Read the model definition and answer for the solid it produces. Units are mm, in the model's axes. A direction names the side the tool comes from. Coordinates: 2 decimals unless noted, no trailing zeros. Order: outer loops, then holes, each group sorted by start corner. A loop starts at its lowest first (then second) coordinate and runs counter-clockwise, first axis right, second up.
```python
from build123d import *

# Parameters (mm, degrees)
S_BOX1_W        = 30.8
S_BOX1_H        = 34.5
BOSS_1_DEPTH    = 2.5
S_BOX2_W        = 30.8
S_BOX2_H        = 34.5
BOSS_2_DEPTH    = 2.5
S_BOX3_W        = 2.5
S_BOX3_H        = 34.5
BOSS_3_DEPTH    = 51.4
S_BOX4_W        = 2.5
S_BOX4_H        = 34.5
BOSS_4_DEPTH    = 51.4
S_BOX5_W        = 30.8
S_BOX5_H        = 3
BOSS_5_DEPTH    = 51.4
S_BOX6_W        = 2.5
S_BOX6_H        = 34.5
BOSS_6_DEPTH    = 30.8
S_BOX7_W        = 2.5
S_BOX7_H        = 34.5
BOSS_7_DEPTH    = 30.8
S_BOX8_W        = 51.4
S_BOX8_H        = 34.5
BOSS_8_DEPTH    = 2.5
S_BOX9_W        = 51.4
S_BOX9_H        = 34.5
BOSS_9_DEPTH    = 2.5
S_BOX10_W       = 51.4
S_BOX10_H       = 3
BOSS_10_DEPTH   = 30.8
BOSS_11_DEPTH   = 34.5
S_CYL12_R       = 3.5
BOSS_12_DEPTH   = 7.7
S_HOLE13_R      = 10.5
HOLE_13_DEPTH   = 3.2
S_CUT14_W       = 19.4
S_CUT14_H       = 3.15
POCKET_14_DEPTH = 19.5
S_CUT15_W       = 16.4
S_CUT15_H       = 3.15
POCKET_15_DEPTH = 8.3
S_CUT16_W       = 7
S_CUT16_H       = 3.15
POCKET_16_DEPTH = 11
S_HOLE17_R      = 1.1
HOLE_17_DEPTH   = 3.2
S_HOLE18_R      = 1.1
HOLE_18_DEPTH   = 3.2
S_HOLE19_R      = 1.1
HOLE_19_DEPTH   = 3.2
S_HOLE20_R      = 1.1
HOLE_20_DEPTH   = 3.2
S_HOLE21_R      = 10.5
HOLE_21_DEPTH   = 3.2
S_CUT22_W       = 19.5
S_CUT22_H       = 3.15
POCKET_22_DEPTH = 19.4
S_CUT23_W       = 8.3
S_CUT23_H       = 3.15
POCKET_23_DEPTH = 16.4
S_CUT24_W       = 11
S_CUT24_H       = 3.15
POCKET_24_DEPTH = 7
S_HOLE25_R      = 1.1
HOLE_25_DEPTH   = 3.2
S_HOLE26_R      = 1.1
HOLE_26_DEPTH   = 3.2
S_HOLE27_R      = 1.1
HOLE_27_DEPTH   = 3.2
S_HOLE28_R      = 1.1
HOLE_28_DEPTH   = 3.2


with BuildPart() as part:
    # S_box1 → Boss_1 (new body)
    with BuildSketch(Plane.XY.offset(-38.2)):
        with Locations((0, -20.15)):
            Rectangle(S_BOX1_W, S_BOX1_H)
    extrude(amount=BOSS_1_DEPTH)



with BuildPart() as body_2:
    # S_box2 → Boss_2 (new body)
    with BuildSketch(Plane.XY.offset(10.7)):
        with Locations((0, -20.15)):
            Rectangle(S_BOX2_W, S_BOX2_H)
    extrude(amount=BOSS_2_DEPTH)


with BuildPart() as part_1:
    add(part.part)

    add(body_2.part)  # Boss_3 merges body 2
    # S_box3 → Boss_3 (add)
    with BuildSketch(Plane.XY.offset(-38.2)):
        with Locations((-14.15, -20.15)):
            Rectangle(S_BOX3_W, S_BOX3_H)
    extrude(amount=BOSS_3_DEPTH)

    # S_box4 → Boss_4 (add)
    with BuildSketch(Plane.XY.offset(-38.2)):
        with Locations((14.15, -20.15)):
            Rectangle(S_BOX4_W, S_BOX4_H)
    extrude(amount=BOSS_4_DEPTH)

    # S_box5 → Boss_5 (add)
    with BuildSketch(Plane.XY.offset(-38.2)):
        with Locations((0, -35.9)):
            Rectangle(S_BOX5_W, S_BOX5_H)
    extrude(amount=BOSS_5_DEPTH)

    # S_box6 → Boss_6 (add)
    with BuildSketch(Plane.XY.offset(-67.4)):
        with Locations((-11.95, -20.85)):
            Rectangle(S_BOX6_W, S_BOX6_H)
    extrude(amount=BOSS_6_DEPTH)



with BuildPart() as body_2_2:
    # S_box7 → Boss_7 (new body)
    with BuildSketch(Plane.XY.offset(-67.4)):
        with Locations((36.95, -20.85)):
            Rectangle(S_BOX7_W, S_BOX7_H)
    extrude(amount=BOSS_7_DEPTH)


with BuildPart() as part_2:
    add(part_1.part)

    add(body_2_2.part)  # Boss_8 merges body 2 2
    # S_box8 → Boss_8 (add)
    with BuildSketch(Plane.XY.offset(-67.4)):
        with Locations((12.5, -20.85)):
            Rectangle(S_BOX8_W, S_BOX8_H)
    extrude(amount=BOSS_8_DEPTH)

    # S_box9 → Boss_9 (add)
    with BuildSketch(Plane.XY.offset(-39.1)):
        with Locations((12.5, -20.85)):
            Rectangle(S_BOX9_W, S_BOX9_H)
    extrude(amount=BOSS_9_DEPTH)

    # S_box10 → Boss_10 (add)
    with BuildSketch(Plane.XY.offset(-67.4)):
        with Locations((12.5, -5.1)):
            Rectangle(S_BOX10_W, S_BOX10_H)
    extrude(amount=BOSS_10_DEPTH)

    # S_prism11 → Boss_11 (add)
    with BuildSketch(Plane(origin=(0, -37.4, 0), x_dir=(1, 0, 0), z_dir=(0, 1, 0))):
        with BuildLine():
            Line((-15.45, -10.75), (15.45, -10.75))
            Line((15.45, -10.75), (15.45, -11.2))
            ThreePointArc((15.45, -11.2), (13.6926, -15.4426), (9.45, -17.2))
            Line((9.45, -17.2), (-9.45, -17.2))
            ThreePointArc((-9.45, -17.2), (-13.6926, -15.4426), (-15.45, -11.2))
            Line((-15.45, -11.2), (-15.45, -10.75))
        make_face()
    extrude(amount=BOSS_11_DEPTH)

    # S_cyl12 → Boss_12 (add)
    with BuildSketch(Plane(origin=(0, -44.2, 0), x_dir=(1, 0, 0), z_dir=(0, 1, 0))):
        with Locations(Location((13, 17, 0), (0, 0, 46.708192407))):
            Circle(S_CYL12_R)
    extrude(amount=BOSS_12_DEPTH)

    # S_hole13 → Hole_13 (cut)
    with BuildSketch(Plane(origin=(0, -37.5, 0), x_dir=(1, 0, 0), z_dir=(0, 1, 0))):
        with Locations(Location((0, 0, 0), (0, 0, 90))):
            Circle(S_HOLE13_R)
    extrude(amount=HOLE_13_DEPTH, mode=Mode.SUBTRACT)

    # S_cut14 → Pocket_14 (cut)
    with BuildSketch(Plane.XY.offset(-30.4)):
        with Locations((0, -35.925)):
            Rectangle(S_CUT14_W, S_CUT14_H)
    extrude(amount=POCKET_14_DEPTH, mode=Mode.SUBTRACT)

    # S_cut15 → Pocket_15 (cut)
    with BuildSketch(Plane.XY.offset(-38.7)):
        with Locations((0, -35.925)):
            Rectangle(S_CUT15_W, S_CUT15_H)
    extrude(amount=POCKET_15_DEPTH, mode=Mode.SUBTRACT)

    # S_cut16 → Pocket_16 (cut)
    with BuildSketch(Plane.XY.offset(-11)):
        with Locations((0, -35.925)):
            Rectangle(S_CUT16_W, S_CUT16_H)
    extrude(amount=POCKET_16_DEPTH, mode=Mode.SUBTRACT)

    # S_hole17 → Hole_17 (cut)
    with BuildSketch(Plane(origin=(0, -37.5, 0), x_dir=(1, 0, 0), z_dir=(0, 1, 0))):
        with Locations(Location((-10.25, 8.3, 0), (0, 0, 90))):
            Circle(S_HOLE17_R)
    extrude(amount=HOLE_17_DEPTH, mode=Mode.SUBTRACT)

    # S_hole18 → Hole_18 (cut)
    with BuildSketch(Plane(origin=(0, -37.5, 0), x_dir=(1, 0, 0), z_dir=(0, 1, 0))):
        with Locations(Location((10.25, 8.3, 0), (0, 0, 90))):
            Circle(S_HOLE18_R)
    extrude(amount=HOLE_18_DEPTH, mode=Mode.SUBTRACT)

    # S_hole19 → Hole_19 (cut)
    with BuildSketch(Plane(origin=(0, -37.5, 0), x_dir=(1, 0, 0), z_dir=(0, 1, 0))):
        with Locations(Location((-10.25, 32.75, 0), (0, 0, 90))):
            Circle(S_HOLE19_R)
    extrude(amount=HOLE_19_DEPTH, mode=Mode.SUBTRACT)

    # S_hole20 → Hole_20 (cut)
    with BuildSketch(Plane(origin=(0, -37.5, 0), x_dir=(1, 0, 0), z_dir=(0, 1, 0))):
        with Locations(Location((10.25, 32.75, 0), (0, 0, 90))):
            Circle(S_HOLE20_R)
    extrude(amount=HOLE_20_DEPTH, mode=Mode.SUBTRACT)

    # S_hole21 → Hole_21 (cut)
    with BuildSketch(Plane(origin=(0, -6.7, 0), x_dir=(1, 0, 0), z_dir=(0, 1, 0))):
        with Locations(Location((0, 52, 0), (0, 0, 90))):
            Circle(S_HOLE21_R)
    extrude(amount=HOLE_21_DEPTH, mode=Mode.SUBTRACT)

    # S_cut22 → Pocket_22 (cut)
    with BuildSketch(Plane.XY.offset(-61.7)):
        with Locations((20.65, -5.075)):
            Rectangle(S_CUT22_W, S_CUT22_H)
    extrude(amount=POCKET_22_DEPTH, mode=Mode.SUBTRACT)

    # S_cut23 → Pocket_23 (cut)
    with BuildSketch(Plane.XY.offset(-60.2)):
        with Locations((34.55, -5.075)):
            Rectangle(S_CUT23_W, S_CUT23_H)
    extrude(amount=POCKET_23_DEPTH, mode=Mode.SUBTRACT)

    # S_cut24 → Pocket_24 (cut)
    with BuildSketch(Plane.XY.offset(-55.5)):
        with Locations((5.5, -5.075)):
            Rectangle(S_CUT24_W, S_CUT24_H)
    extrude(amount=POCKET_24_DEPTH, mode=Mode.SUBTRACT)

    # S_hole25 → Hole_25 (cut)
    with BuildSketch(Plane(origin=(0, -6.7, 0), x_dir=(1, 0, 0), z_dir=(0, 1, 0))):
        with Locations(Location((8.3, 62.25, 0), (0, 0, 90))):
            Circle(S_HOLE25_R)
    extrude(amount=HOLE_25_DEPTH, mode=Mode.SUBTRACT)

    # S_hole26 → Hole_26 (cut)
    with BuildSketch(Plane(origin=(0, -6.7, 0), x_dir=(1, 0, 0), z_dir=(0, 1, 0))):
        with Locations(Location((8.3, 41.75, 0), (0, 0, 90))):
            Circle(S_HOLE26_R)
    extrude(amount=HOLE_26_DEPTH, mode=Mode.SUBTRACT)

    # S_hole27 → Hole_27 (cut)
    with BuildSketch(Plane(origin=(0, -6.7, 0), x_dir=(1, 0, 0), z_dir=(0, 1, 0))):
        with Locations(Location((32.75, 62.25, 0), (0, 0, 90))):
            Circle(S_HOLE27_R)
    extrude(amount=HOLE_27_DEPTH, mode=Mode.SUBTRACT)

    # S_hole28 → Hole_28 (cut)
    with BuildSketch(Plane(origin=(0, -6.7, 0), x_dir=(1, 0, 0), z_dir=(0, 1, 0))):
        with Locations(Location((32.75, 41.75, 0), (0, 0, 90))):
            Circle(S_HOLE28_R)
    extrude(amount=HOLE_28_DEPTH, mode=Mode.SUBTRACT)


solid = part_2.part
```
1) A cutting plane is placed at D-D, the plane x = 0. Determine the outline of the cut face in (y, z), and give its area (3 significant figures).
A:
outline: (-38.1, -67.4) - (-3.6, -67.4) - (-3.6, -62.5) - (-6.6, -62.5) - (-6.6, -64.9) - (-38.1, -64.9) - close; (-38.1, -39.1) - (-6.6, -39.1) - (-6.6, -41.5) - (-3.6, -41.5) - (-3.6, -38.2) - (-2.9, -38.2) - (-2.9, -35.7) - (-34.35, -35.7) - (-34.35, -38.7) - (-37.5, -38.7) - (-37.5, -36.6) - (-38.1, -36.6) - close; (-37.4, 10.5) - (-34.4, 10.5) - (-34.4, 10.7) - (-2.9, 10.7) - (-2.9, 17.2) - (-37.4, 17.2) - close
area: 435 mm2
2) Flat-ended cylindrical pins translate along their axes: pin 1 Ø5 at (y, z) = (-30.5, -8.5) entering from -X; pin 2 Ø24.5 at (x, z) = (1, -59.5) entering from +Y; pin 3 Ø12 at (y, z) = (-34.5, -26.5) entering from +X. Find the tip coordinate at first contact, or state that the pin passes through.
A:
pin 1: stops at x = -15.4
pin 2: stops at y = -3.6
pin 3: stops at x = 15.4
3) A cutting plane is placed at B-B, the plane x = 32.75. Determine the outline of the cut face in (y, z), and give its area (4 significant figures).
A:
outline: (-38.1, -67.4) - (-3.6, -67.4) - (-3.6, -63.35) - (-6.6, -63.35) - (-6.6, -64.9) - (-38.1, -64.9) - close; (-38.1, -39.1) - (-6.6, -39.1) - (-6.6, -40.65) - (-3.6, -40.65) - (-3.6, -36.6) - (-38.1, -36.6) - close; (-6.6, -61.15) - (-3.6, -61.15) - (-3.6, -60.2) - (-6.6, -60.2) - close; (-6.6, -43.8) - (-3.6, -43.8) - (-3.6, -42.85) - (-6.6, -42.85) - close
area: 187.5 mm2
4) Straight lines are drawn through the part: line 1 (Z direction, x = -2, y = -10.5); line 2 (X direction, y = -35.15, z = -32.75); line 3 (Z direction, x = 24, y = -30). For each, find the intervals that lie inside material, in ascending order.
A:
line 1: z = -67.4 to -64.9, -39.1 to -35.7, 10.7 to 17.2
line 2: x = -15.4 to -11.35, -9.15 to -8.2, 8.2 to 9.15, 11.35 to 15.4
line 3: z = -67.4 to -64.9, -39.1 to -36.6
5) A cutting plane is placed at A-A, the plane y = -28.5. Determine the outline of the cut face in (x, z).
A:
outline: (-15.45, 10.75) - (-15.4, 10.75) - (-15.4, -38.2) - (-13.2, -38.2) - (-13.2, -67.4) - (38.2, -67.4) - (38.2, -36.6) - (15.4, -36.6) - (15.4, 10.75) - (15.45, 10.75) - (15.45, 11.2) arc R6 ccw to (15.4, 11.97) - (15.4, 13.2) - (15.11, 13.2) arc R6 ccw to (9.45, 17.2) - (-9.45, 17.2) arc R6 ccw to (-15.11, 13.2) - (-15.4, 13.2) - (-15.4, 11.97) arc R6 ccw to (-15.45, 11.2) - close; hole (-12.9, -35.7) - (12.9, -35.7) - (12.9, 10.7) - (-12.9, 10.7) - close; hole (-10.7, -64.9) - (35.7, -64.9) - (35.7, -39.1) - (-10.7, -39.1) - close
6) Determine the mould class of faces 1 (the flat face through (0, -36, -38.7)), 2 (the flat face through (13, -44.2, -17)), 3 (the flat face through (12, -22, -39.1)) for opening direction Y: pulls with the +Y half, pulls with the -Y half, needs draft (parallel to the pull), parting line crosses it, or undercut.
A:
face 1: undercut
face 2: pulls with the -Y half
face 3: needs draft
7) Which of the six approach directions +Z, -Z, +X, -X, +Y, -Y give full straight-line access (tool end or side, diameter ignored) to faces 4 (the cylindrical face through (16.193, -40.404, -18.434)), 5 (the flat face through (14, -2.9, -4)), 6 (the flat face through (-7.7, -34.4, -7.5)), 7 (the flat face through (34, -5, -60.2))?
A:
face 4: -Y
face 5: +Z, -Z, +X, -X, +Y
face 6: +Y
face 7: +X, +Y
8) A cutting plane is placed at C-C, the plane z = -26. Determine the outline of the cut face in (x, y), and give its area (3 significant figures).
A:
outline: (-15.4, -37.4) - (-9.7, -37.4) - (-9.7, -34.4) - (-12.9, -34.4) - (-12.9, -2.9) - (-15.4, -2.9) - close; (9.7, -37.4) - (15.4, -37.4) - (15.4, -2.9) - (12.9, -2.9) - (12.9, -34.4) - (9.7, -34.4) - close
area: 192 mm2
